from build123d import *

# Parameters (mm, degrees)
CUT_EXTRUDE_1_DEPTH = 2


with BuildPart() as part:
    # Эскиз1 → Повернуть1 (revolve)
    with BuildSketch(Plane.XY, mode=Mode.PRIVATE) as revolve_1_sk:
        with BuildLine():
            Line((0, 0), (44, 0))
            Line((44, 0), (44, 3))
            Line((44, 3), (4, 3))
            Line((4, 3), (4, 6))
            Line((4, 6), (2.5, 6))
            ThreePointArc((2.5, 6), (0.732233047, 5.267766953), (0, 3.5))
            Line((0, 3.5), (0, 0))
        make_face()
    revolve(revolve_1_sk.sketch.rotate(Axis((-40.27641129, 0, 0), (1, 0, 0)), 90), axis=Axis((-40.27641129, 0, 0), (1, 0, 0)))

    # Эскиз2 → Вырез-Вытянуть1 (cut)
    with BuildSketch(Plane.ZY):
        Polygon((-0.5, -6.861954459), (0.5, -6.861954459), (0.5, -0.5), (7.705566097, -0.5), (7.705566097, 0.5), (0.5, 0.5), (0.5, 7.070683112), (-0.5, 7.070683112), (-0.5, 0.5), (-7.496837445, 0.5), (-7.496837445, -0.5), (-0.5, -0.5), align=None)
    extrude(amount=-CUT_EXTRUDE_1_DEPTH, mode=Mode.SUBTRACT)


solid = part.part
Work out the finished part from the listing and answer in its coordinate system (mm). A direction names the side the tool comes from. Give positions to 0.01 mm unless a question says otherwise; leave off trailing zeros. Loops run counter-clockwise (first coordinate to the right, second up) from the corner with the lowest first, then second, coordinate; pieces in that order, holes last. Notation, with made-up numbers: (-32.75, -13.5) - (6.25, -13.5) arc R12 cw to (6.25, 4.5) - close; hole circle Ø11 at (-12.5, -20.5). An arc over 180 degrees is marked (long way). Answer in a Markdown table with one row per item. Add a question column.
Q1. Each of these flat-tipped pins is pushed along its axis until it touches: P1, Ø6, axis at x = 10, z = -3, coming from the +Y side; P2, Ø1, axis at x = 1.5, y = -4, coming from the +Z side; P3, Ø4, axis at x = 39, z = -2, coming from the -Y side. Where does it stop, or does it pass through?
Q2. Consider line 1 along X through (y, z) = (-3.25, 0.75); line 2 along Y through (x, z) = (33, 0.75); line 3 along X through (y, z) = (-4, -2.5). Determine where each line is inside the solid, lowest interval first.
Q3. A tool of negligible diameter and unlimited length cuts with its end or side. For faces 1 (the flat face through (1, 0.5, 3)), 2 (the flat face through (1, -3, 0.5)), 3 (the flat face through (44, 0, 0)), 4 (the flat face through (0, -2, -2)), 5 (the flat face through (4, -3, -1)), from which of +Z, -Z, +X, -X, +Y, -Y can it reach the whole face along a straight path? Write none if from no direction.
Q4. The part is cut by section C-C (x = 29.5). Determine the outline of the cut face in (y, z), and give its area (3 significant figures).
Q5. The part is cut by section A-A (y = 0). Determine the outline of the cut face in (x, z).
Q6. Determine the mould class of faces 6 (the flat face through (2, 0, 0)), 7 (the flat face through (1, -0.5, 3)), 8 (the cylindrical face through (23.72, -0.9, 2.86)), 9 (the flat face through (1, 3, 0.5)) for opening direction Z: released by +Z, released by -Z, zero draft, split by the parting line, or undercut.
Solution:
| question | item | result |
|---|---|---|
| 1 | P1 | stops at y = 3 |
| 1 | P2 | stops at z = 4.68 |
| 1 | P3 | stops at y = -3 |
| 2 | line 1 | x = 0 to 4 |
| 2 | line 2 | y = -2.9 to 2.9 |
| 2 | line 3 | x = 0.32 to 4 |
| 3 | face 1 | +Z, -Z, -X |
| 3 | face 2 | -X, +Y, -Y |
| 3 | face 3 | +Z, -Z, +X, +Y, -Y |
| 3 | face 4 | +Z, -Z, -X, +Y, -Y |
| 3 | face 5 | +X |
| 4 | outline | circle Ø6 at (0, 0) |
| 4 | area | 28.3 mm² |
| 5 | outline | (2, -5.95) arc R2.5 ccw to (2.5, -6) - (4, -6) - (4, -3) - (44, -3) - (44, 3) - (4, 3) - (4, 6) - (2.5, 6) arc R2.5 ccw to (2, 5.95) - close |
| 6 | face 6 | undercut |
| 6 | face 7 | zero draft |
| 6 | face 8 | split by the parting line |
| 6 | face 9 | undercut |
